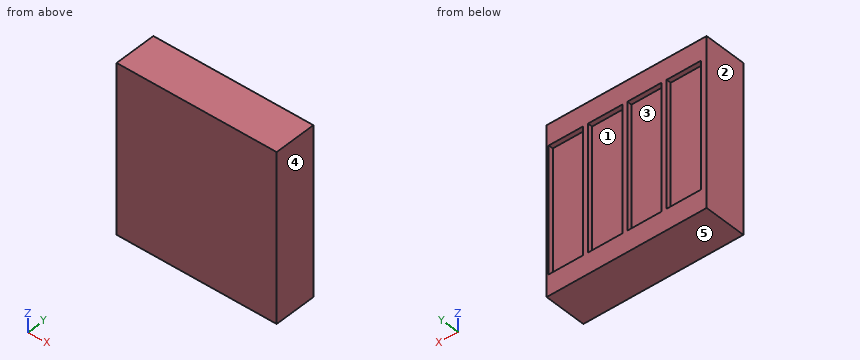
Autodesk Fusion 360 part; units mm, degrees
sketch "スケッチ1" plane through (0, 0, 0) normal (0, 1, 0) x (1, 0, 0)
  line L0 (0, 0) -> (-114, 0)
  line L1 (-114, 0) -> (-114, 120)
  line L2 (-114, 120) -> (0, 120)
  line L3 (0, 120) -> (0, 0)
  dimension "d1" = 114
  dimension "d2" = 120
extrude "押し出し1" add sketch "スケッチ1" along normal blind 40
sketch "スケッチ2" plane through (0, 40, 0) normal (0, 1, 0) x (-1, 0, 0)
  line L0 (0, -120) -> (114, -120)
  line L1 (114, -120) -> (114, 0)
  line L2 (114, 0) -> (0, 0)
  line L3 (0, 0) -> (0, -120)
  line L4 (0, -105) -> (1.5, -105)
  line L5 (1.5, -105) -> (1.5, -15)
  line L6 (1.5, -15) -> (0, -15)
  line L7 (0, -15) -> (0, -105)
  line L8 (1.5, -105) -> (26, -105)
  line L9 (26, -105) -> (26, -15)
  line L10 (26, -15) -> (1.5, -15)
  line L11 (1.5, -15) -> (1.5, -105)
  line L12 (26, -105) -> (29.5, -105)
  line L13 (29.5, -105) -> (29.5, -15)
  line L14 (29.5, -15) -> (26, -15)
  line L15 (26, -15) -> (26, -105)
  line L16 (29.5, -105) -> (54, -105)
  line L17 (54, -105) -> (54, -15)
  line L18 (54, -15) -> (29.5, -15)
  line L19 (29.5, -15) -> (29.5, -105)
  line L20 (54, -105) -> (57.5, -105)
  line L21 (57.5, -105) -> (57.5, -15)
  line L22 (57.5, -15) -> (54, -15)
  line L23 (54, -15) -> (54, -105)
  line L24 (57.5, -105) -> (82, -105)
  line L25 (82, -105) -> (82, -15)
  line L26 (82, -15) -> (57.5, -15)
  line L27 (57.5, -15) -> (57.5, -105)
  line L28 (82, -105) -> (85.5, -105)
  line L29 (85.5, -105) -> (85.5, -15)
  line L30 (85.5, -15) -> (82, -15)
  line L31 (82, -15) -> (82, -105)
  line L32 (85.5, -105) -> (110, -105)
  line L33 (110, -105) -> (110, -15)
  line L34 (110, -15) -> (85.5, -15)
  line L35 (85.5, -15) -> (85.5, -105)
  line L36 (110, -105) -> (114, -105)
  line L37 (114, -105) -> (114, -15)
  line L38 (114, -15) -> (110, -15)
  line L39 (110, -15) -> (110, -105)
  dimension "d5" = 1.5
  dimension "d6" = 90
  dimension "d7" = 24.5
  dimension "d8" = 90
  dimension "d9" = 3.5
  dimension "d10" = 90
  dimension "d11" = 24.5
  dimension "d12" = 90
  dimension "d13" = 3.5
  dimension "d14" = 90
  dimension "d15" = 24.5
  dimension "d16" = 90
  dimension "d17" = 3.5
  dimension "d18" = 90
  dimension "d19" = 24.5
  dimension "d20" = 90
  dimension "d21" = 4
  dimension "d22" = 90
extrude "押し出し2" cut sketch "スケッチ2" against normal blind 3 contours L29 L32 L33 L34 L35 L39
sketch "スケッチ3" plane through (0, 40, 0) normal (0, 1, 0) x (-1, 0, 0)
  line L0 (110, -105) -> (85.5, -105)
  line L1 (85.5, -105) -> (85.5, -15)
  line L2 (85.5, -15) -> (110, -15)
  line L3 (110, -15) -> (110, -105)
  line L4 (0, -120) -> (114, -120)
  line L5 (114, -120) -> (114, 0)
  line L6 (114, 0) -> (0, 0)
  line L7 (0, 0) -> (0, -120)
  line L8 (0, -105) -> (1.5, -105)
  line L9 (1.5, -105) -> (1.5, -15)
  line L10 (1.5, -15) -> (0, -15)
  line L11 (0, -15) -> (0, -105)
  line L12 (1.5, -105) -> (26, -105)
  line L13 (26, -105) -> (26, -15)
  line L14 (26, -15) -> (1.5, -15)
  line L15 (1.5, -15) -> (1.5, -105)
  dimension "d25" = 1.5
  dimension "d26" = 90
  dimension "d27" = 24.5
  dimension "d28" = 90
extrude "押し出し3" cut sketch "スケッチ3" against normal blind 3 contours L9 L12 L13 L14 L15
extrude "押し出し4" cut 1 faces at (-93.6667, 37, -45) along direction (0, -1, 0) blind 0.3
extrude "押し出し5" cut 1 faces at (-9.6667, 37, -45) along direction (0, -1, 0) blind 0.3
sketch "スケッチ4" plane through (0, 40, 0) normal (0, 1, 0) x (-1, 0, 0)
  line L0 (26, -105) -> (1.5, -105)
  line L1 (1.5, -105) -> (1.5, -15)
  line L2 (1.5, -15) -> (26, -15)
  line L3 (26, -15) -> (26, -105)
  line L4 (110, -105) -> (85.5, -105)
  line L5 (85.5, -105) -> (85.5, -15)
  line L6 (85.5, -15) -> (110, -15)
  line L7 (110, -15) -> (110, -105)
  line L8 (0, -120) -> (114, -120)
  line L9 (114, -120) -> (114, 0)
  line L10 (114, 0) -> (0, 0)
  line L11 (0, 0) -> (0, -120)
  line L12 (26, -105) -> (29.5, -105)
  line L13 (29.5, -105) -> (29.5, -15)
  line L14 (29.5, -15) -> (26, -15)
  line L15 (26, -15) -> (26, -105)
  line L16 (29.5, -105) -> (54, -105)
  line L17 (54, -105) -> (54, -15)
  line L18 (54, -15) -> (29.5, -15)
  line L19 (29.5, -15) -> (29.5, -105)
  dimension "d35" = 3.5
  dimension "d36" = 90
  dimension "d37" = 24.5
  dimension "d38" = 90
extrude "押し出し6" cut sketch "スケッチ4" against normal blind 3.3 contours L13 L16 L17 L18 L19
sketch "スケッチ5" plane through (0, 40, 0) normal (0, 1, 0) x (-1, 0, 0)
  line L0 (54, -105) -> (29.5, -105)
  line L1 (29.5, -105) -> (29.5, -15)
  line L2 (29.5, -15) -> (54, -15)
  line L3 (54, -15) -> (54, -105)
  line L4 (26, -105) -> (1.5, -105)
  line L5 (1.5, -105) -> (1.5, -15)
  line L6 (1.5, -15) -> (26, -15)
  line L7 (26, -15) -> (26, -105)
  line L8 (110, -105) -> (85.5, -105)
  line L9 (85.5, -105) -> (85.5, -15)
  line L10 (85.5, -15) -> (110, -15)
  line L11 (110, -15) -> (110, -105)
  line L12 (0, -120) -> (114, -120)
  line L13 (114, -120) -> (114, 0)
  line L14 (114, 0) -> (0, 0)
  line L15 (0, 0) -> (0, -120)
  line L16 (54, -105) -> (57.5, -105)
  line L17 (57.5, -105) -> (57.5, -15)
  line L18 (57.5, -15) -> (54, -15)
  line L19 (54, -15) -> (54, -105)
  line L20 (57.5, -105) -> (82, -105)
  line L21 (82, -105) -> (82, -15)
  line L22 (82, -15) -> (57.5, -15)
  line L23 (57.5, -15) -> (57.5, -105)
  dimension "d41" = 3.5
  dimension "d42" = 90
  dimension "d43" = 24.5
  dimension "d44" = 90
extrude "押し出し7" cut sketch "スケッチ5" against normal blind 3.3 contours L17 L20 L21 L22 L23
extrude "押し出し8" cut 4 faces at (-93.6667, 36.7, -45) (-65.6667, 36.7, -45) (-37.6667, 36.7, -45) (-9.6667, 36.7, -45) along direction (0, -1, 0) blind 10
extrude "押し出し9" cut 1 faces at (-57.1667, 40, -5) along direction (0, -1, 0) blind 10
Build history of the part. All positions in model axes, mm. Face numbers are marked on the shaded views. A direction names the side the tool comes from. Give positions to 0.01 mm unless a question says otherwise; leave off trailing zeros. Loops run counter-clockwise (first coordinate to the right, second up) from the corner with the lowest first, then second, coordinate; pieces in that order, holes last.
1) Drop a flat-ended pin along its axis: P1, Ø12, axis at x = -98, z = -94, coming from the +Y side. Give the stop position or say it passes through.
Values follow:
P1: stops at y = 26.7
2) Two-plate mould, pull along X, no slides. Class the marked faces 3, 4 and 5: released by +X, released by -X, zero draft, split by the parting line, or undercut.
Values follow:
face 3: undercut
face 4: released by +X
face 5: zero draft
3) Probe line 1 along X through (y, z) = (28, -83); line 2 along Z through (x, y) = (-38.5, 26.75); line 3 along Y through (x, z) = (-74, -48.5). List the from-to ranges inside material, lowest first.
Values follow:
line 1: x = -114 to -110, -85.5 to -82, -57.5 to -54, -29.5 to -26, -1.5 to 0
line 2: z = -120 to -105, -15 to 0
line 3: y = 0 to 26.7
4) Band-saw the part on A-A on z = -67. List the corners of the cut face in (x, y).
Values follow:
outline: (-114, 0) - (0, 0) - (0, 30) - (-1.5, 30) - (-1.5, 26.7) - (-26, 26.7) - (-26, 30) - (-29.5, 30) - (-29.5, 26.7) - (-54, 26.7) - (-54, 30) - (-57.5, 30) - (-57.5, 26.7) - (-82, 26.7) - (-82, 30) - (-85.5, 30) - (-85.5, 26.7) - (-110, 26.7) - (-110, 30) - (-114, 30) - close
5) Band-saw the part on B-B on x = -13. List the corners of the cut face in (y, z).
Values follow:
outline: (0, -120) - (30, -120) - (30, -105) - (26.7, -105) - (26.7, -15) - (30, -15) - (30, 0) - (0, 0) - close
6) 3-axis set-ups, long thin cutter, end or side, ignore diameter. For the marked faces 1 and 2: which of +Z, -Z, +X, -X, +Y, -Y reach the whole face in a straight line?
Values follow:
face 1: +Y
face 2: +Z, -Z, -X, +Y, -Y
